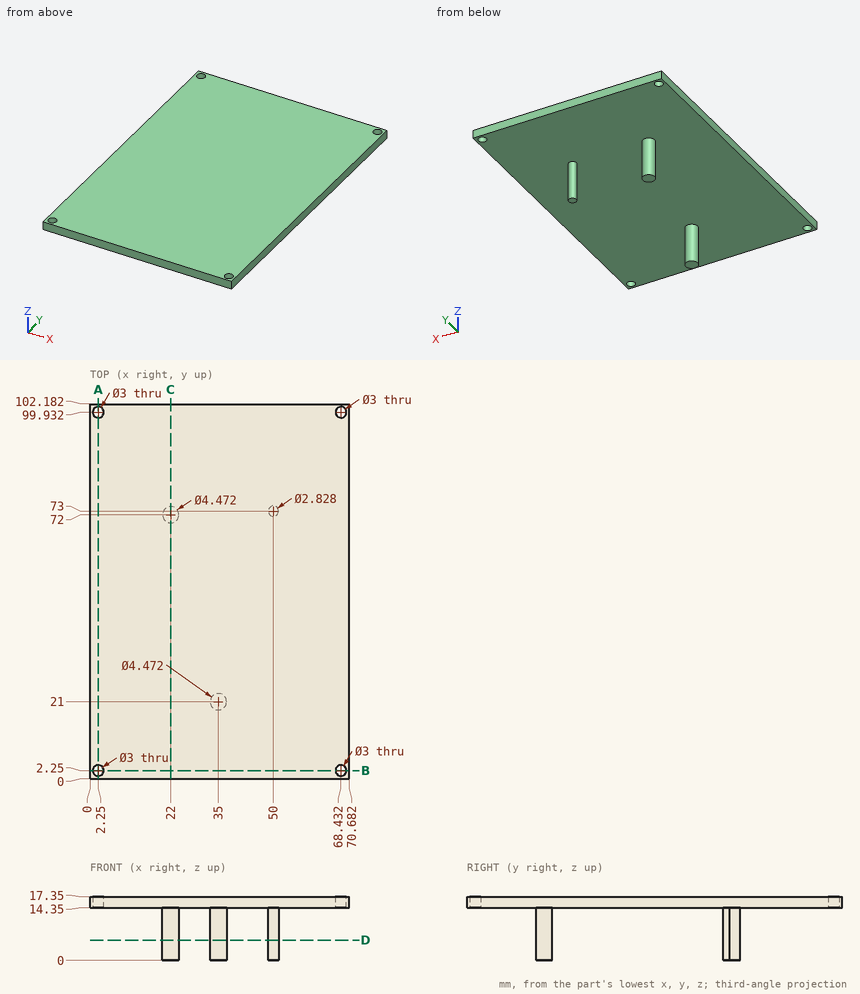
Study the drawing (mm; zero at the part's minimum x, y, z) and answer. Give positions to 0.01 mm unless a question says otherwise; leave off trailing zeros. Loops run counter-clockwise (first coordinate to the right, second up) from the corner with the lowest first, then second, coordinate; pieces in that order, holes last. Notation, with made-up numbers: M 68,53 L 92,53 A35 ccw 92,89 Z; hole C 87,37 d11. An arc over 180 degrees is marked long. One line per item, written item: value.
1. Section A-A on x = 2.25 is taken. Determine the outline of the cut face in (y, z).
Found:
outline: M 0,14.35 L 0.75,14.35 L 0.75,17.35 L 0,17.35 Z; M 3.75,14.35 L 98.43,14.35 L 98.43,17.35 L 3.75,17.35 Z; M 101.43,14.35 L 102.18,14.35 L 102.18,17.35 L 101.43,17.35 Z
2. Each of these flat-tipped pins is pushed along its axis until it touches: P1, Ø2, axis at x = 21.5, z = 10.5, coming from the +Y side; P2, Ø4, axis at x = 68.43, y = 99.93, coming from the -Z side. Where does it stop, or does it pass through?
Found:
P1: y = 74.24
P2: z = 14.35
3. Section C-C on x = 22 is taken. Determine the outline of the cut face in (y, z).
Found:
outline: M 0,14.35 L 69.76,14.35 L 69.76,0 L 74.24,0 L 74.24,14.35 L 102.18,14.35 L 102.18,17.35 L 0,17.35 Z
4. Section D-D on z = 5.5 is taken. Determine the outline of the cut face in (x, y) (1 decimal), plus the area to 3 significant figures.
Found:
outline: C 22,72 d4.5; C 35,21 d4.5; C 50,73 d2.8
area: 37.7 mm^2
5. Find the intervals of material crossed by probe 1 along Y at (x, z) = (2.25, 16.3); probe 2 along X at (y, z) = (2.25, 16.4); probe 3 along Z at (x, y) = (28, 73.5), in increasing order.
Found:
probe 1: 0 to 0.75, 3.75 to 98.43, 101.43 to 102.18
probe 2: 0 to 0.75, 3.75 to 66.93, 69.93 to 70.68
probe 3: 14.35 to 17.35
6. Section B-B on y = 2.25 is taken. Determine the outline of the cut face in (x, z), plus the area to 3 significant figures.
Found:
outline: M 0,14.35 L 0.75,14.35 L 0.75,17.35 L 0,17.35 Z; M 3.75,14.35 L 66.93,14.35 L 66.93,17.35 L 3.75,17.35 Z; M 69.93,14.35 L 70.68,14.35 L 70.68,17.35 L 69.93,17.35 Z
area: 194 mm^2
